from build123d import *

# Parameters (mm, degrees)
SKETCH1_W           = 56
SKETCH1_H           = 56
BOSS_EXTRUDE1_DEPTH = 11.5
SKETCH2_W           = 9
SKETCH2_H           = 9
CUT_EXTRUDE1_DEPTH  = 11.5
CIRPATTERN1_COUNT   = 4
FILLET1_R           = 5
FILLET2_R           = 2
SKETCH3_R           = 6
CUT_EXTRUDE2_DEPTH  = 11.5


with BuildPart() as part:
    # Sketch1 → Boss-Extrude1 (new body)
    with BuildSketch(Plane.XY):
        Rectangle(SKETCH1_W, SKETCH1_H)
    extrude(amount=BOSS_EXTRUDE1_DEPTH)

    # Sketch2 → Cut-Extrude1 (cut)
    with BuildSketch(Plane.XY.offset(11.5)):
        with Locations((23.5, 23.5)):
            Rectangle(SKETCH2_W, SKETCH2_H)
    cut_extrude1 = extrude(amount=-CUT_EXTRUDE1_DEPTH, mode=Mode.SUBTRACT)

    # CirPattern1: Cut-Extrude1 ×4 about axis
    cirpattern1_axis = Axis((0, 0, 0), (0, 0, 1))
    for i in range(1, CIRPATTERN1_COUNT):
        add(cut_extrude1.rotate(cirpattern1_axis, i * 360 / CIRPATTERN1_COUNT), mode=Mode.SUBTRACT)

    # Fillet1
    fillet1_edges = [part.edges().sort_by_distance(p)[0] for p in [
        (19, 19, 5.75),
        (-19, 19, 5.75),
        (-19, -19, 5.75),
        (19, -19, 5.75),
    ]]
    fillet(fillet1_edges, radius=FILLET1_R)

    # Fillet2
    fillet2_edges = [part.edges().sort_by_distance(p)[0] for p in [
        (19, 28, 5.75),
        (28, 19, 5.75),
        (-28, 19, 5.75),
        (-19, 28, 5.75),
        (-19, -28, 5.75),
        (-28, -19, 5.75),
        (28, -19, 5.75),
        (19, -28, 5.75),
    ]]
    fillet(fillet2_edges, radius=FILLET2_R)

    # Sketch3 → Cut-Extrude2 (cut)
    with BuildSketch(Plane.XY.offset(11.5)):
        Circle(SKETCH3_R)
    extrude(amount=-CUT_EXTRUDE2_DEPTH, mode=Mode.SUBTRACT)


solid = part.part
Work out the finished part from the listing and answer in its coordinate system (mm). A direction names the side the tool comes from. Round coordinates to 2 decimals unless told otherwise and drop trailing zeros. Write each loop counter-clockwise with the first axis right and the second up, starting at its lowest first coordinate (ties: lowest second). Pieces come first, ordered by that corner, then holes. Notation, with made-up numbers: (-2.5, 79.25) -> (47.5, 79.25) arc R25 cw to (47.5, 116.25) -> close; hole circle Ø2 at (-9.5, -17.5). An arc over 180 degrees is marked (long way). Answer as CSV lines item,"result". Start each with the question number.
(1) A tool of negligible diameter and unlimited length cuts with its end or side. For faces 1 (the flat face through (25, 19, 6)), 2 (the flat face through (-19, -25, 6)), 3 (the flat face through (-19, 25, 6)), from which of +Z, -Z, +X, -X, +Y, -Y can it reach the whole face along a straight path? Write none if from no direction.
(2) The mould has two halves that part along Y. Classify faces 4 (the flat face through (19, 25, 6)), 5 (the flat face through (0, 28, 6)), 6 (the cylindrical face through (-6, 0, 6)): +Y half, -Y half, draft (parallel to the pull), parting line (faces both ways), or undercut.
(3) Find the intervals of material crossed by probe 1 along Y at (x, z) = (0, 6.75); probe 2 along Y at (x, z) = (-5.5, 4.5); probe 3 along X at (y, z) = (1.5, 4.5), in increasing order.
(4) Each of these flat-tipped pins is pushed along its axis until it touches: pin 1 (3 mm diameter, centred on x = -1, y = 4.5, fed in from +Z); pin 2 (1.6 mm diameter, centred on y = 24.5, z = 7, fed in from +X); pin 3 (0.6 mm diameter, centred on y = -24.5, z = 7.5, fed in from -X); pin 4 (1.6 mm diameter, centred on x = 25, z = 7, fed in from -Y). Where does it stop, or does it pass through?
(5) The part is cut by section A-A, the plane x = 0. Give the vertices of the cut face in (y, z), then the cut area to 3 significant figures.
(6) The part is cut by section D-D, the plane y = -22.5. Give the vertices of the cut face in (x, z).
(7) The part is cut by section C-C, the plane z = 4. Give the vertices of the cut face in (x, y), then the cut area to 3 significant figures.
Output values:
1,face 1,"+Z, -Z, +X, +Y"
1,face 2,"+Z, -Z, -X, -Y"
1,face 3,"+Z, -Z, -X, +Y"
2,face 4,"draft"
2,face 5,"+Y half"
2,face 6,"undercut"
3,probe 1,"y = -28 to -6, 6 to 28"
3,probe 2,"y = -28 to -2.4, 2.4 to 28"
3,probe 3,"x = -28 to -5.81, 5.81 to 28"
4,pin 1,"stops at z = 11.5"
4,pin 2,"stops at x = 19.01"
4,pin 3,"stops at x = -19"
4,pin 4,"stops at y = -19"
5,outline,"(-28, 0) -> (-6, 0) -> (-6, 11.5) -> (-28, 11.5) -> close; (6, 0) -> (28, 0) -> (28, 11.5) -> (6, 11.5) -> close"
5,area,"506 mm²"
6,outline,"(-19.23, 0) -> (19.23, 0) -> (19.23, 11.5) -> (-19.23, 11.5) -> close"
7,outline,"(-28, -17) arc R2 ccw to (-26, -19) -> (-24, -19) arc R5 cw to (-19, -24) -> (-19, -26) arc R2 ccw to (-17, -28) -> (17, -28) arc R2 ccw to (19, -26) -> (19, -24) arc R5 cw to (24, -19) -> (26, -19) arc R2 ccw to (28, -17) -> (28, 17) arc R2 ccw to (26, 19) -> (24, 19) arc R5 cw to (19, 24) -> (19, 26) arc R2 ccw to (17, 28) -> (-17, 28) arc R2 ccw to (-19, 26) -> (-19, 24) arc R5 cw to (-24, 19) -> (-26, 19) arc R2 ccw to (-28, 17) -> close; hole circle Ø12 at (0, 0)"
7,area,"2,710 mm²"
